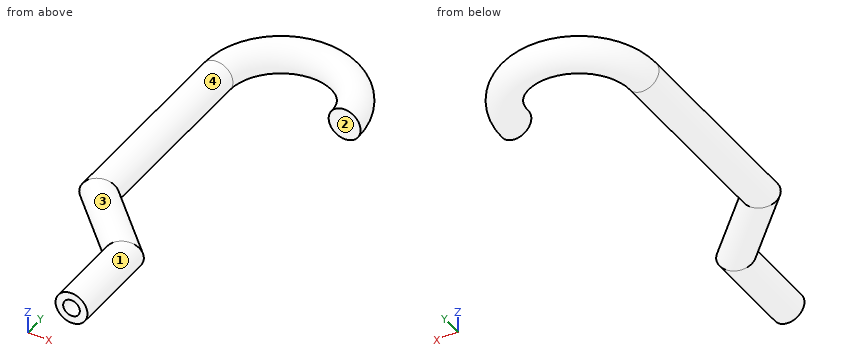
Autodesk Inventor part; units mm, degrees
ref_plane "YZ Plane" through (0, 0, 0) normal (1, 0, 0) x (0, 1, 0)
ref_plane "XZ Plane" through (0, 0, 0) normal (0, 1, 0) x (-1, 0, 0)
ref_plane "XY Plane" through (0, 0, 0) normal (0, 0, 1) x (1, 0, 0)
sketch "Sketch1" plane through (0, 0, 0) normal (0, 0, 1) x (1, 0, 0)
  arc A0 (19.05, 101.6) -> (-19.05, 101.6) centre (0, 101.6) ccw
  line L0 (-19.05, 101.6) -> (-19.05, 44.45)
  line L1 (-19.05, 44.45) -> (0, 25.4)
  line L2 (0, 25.4) -> (0, 0)
  dimension "d1" = 19.05
  dimension "d2" = 45
  dimension "d5" = 25.4
  dimension "d6" = 101.6
sketch "Sketch2" plane through (0, 0, 0) normal (0, 1, 0) x (-1, 0, 0)
  circle A0 centre (0, 0) radius 4.7625
  dimension "d7" = 9.525
sweep "Sweep1" add profiles "Sketch2" path "Sketch1"
sketch "Sketch3" plane through (0, 0, 0) normal (0, -1, 0) x (1, 0, 0)
  point P0 (0, 0)
  point P1 (0, 0)
hole "Hole1" at (0, 0, 0) direction (0, 1, 0) diameter 4.9784 depth 19.05 tip angle 118
Geometry check sheet. Reference: the model listing, model coordinates, mm. Face numbers are marked on the shaded views. Coordinates: 2 decimals unless noted, no trailing zeros.
Item 1: Scan lines: line 1 along X through (y, z) = (5, 0); line 2 along X through (y, z) = (68.5, -0.25). Record each from-to range of solid material in increasing order.
Item 2: Mould release check, pull along Y, two halves, no side actions. Record for the marked faces 1, 2, 3 and 4: released by +Y, released by -Y, zero draft, split by the parting line, or undercut.
Item 3: Depth check by flat-ended pin: pin 1 (4 mm diameter, centred on x = 0, z = 0, fed in from -Y); pin 2 (3 mm diameter, centred on y = 48, z = -2.5, fed in from +X); pin 3 (5 mm diameter, centred on x = 20, z = -1.5, fed in from -Y). Enter the tip coordinate at first touch or a pass-through.
Check sheet entries:
1. line 1: x = -4.76 to -2.49, 2.49 to 4.76
1. line 2: x = -23.81 to -14.29
2. face 1: zero draft
2. face 2: released by -Y
2. face 3: undercut
2. face 4: undercut
3. pin 1: stops at y = 19.34
3. pin 2: stops at x = -14.39
3. pin 3: stops at y = 101.6
